```python
from build123d import *

# Parameters (mm, degrees)
ESQUISSE1_W                                        = 100
ESQUISSE1_H                                        = 150
BOSS_EXTRU_1_DEPTH                                 = 15
ESQUISSE2_W                                        = 25
ESQUISSE2_H                                        = 70
BOSS_EXTRU_2_DEPTH                                 = 60
ENL_V_MAT_EXTRU_1_DEPTH                            = 4.15
CHAMBRAGE_POUR_VIS_T_TE_RONDE_BOMB_E_M_D           = 3.4
CHAMBRAGE_POUR_VIS_T_TE_RONDE_BOMB_E_M_CBORE_D     = 7
CHAMBRAGE_POUR_VIS_T_TE_RONDE_BOMB_E_M_CBORE_DEPTH = 2.4
BOSS_EXTRU_3_DEPTH                                 = 10
CONG_1_R                                           = 7
CONG_2_R                                           = 2


with BuildPart() as part:
    # Esquisse1 → Boss.-Extru.1 (new body)
    with BuildSketch(Plane.XY):
        with Locations((50, 0)):
            Rectangle(ESQUISSE1_W, ESQUISSE1_H)
    extrude(amount=BOSS_EXTRU_1_DEPTH)

    # Esquisse2 → Boss.-Extru.2 (add)
    with BuildSketch(Plane.XY.offset(15)):
        with Locations((-12.5, 0)):
            Rectangle(ESQUISSE2_W, ESQUISSE2_H)
    extrude(amount=-BOSS_EXTRU_2_DEPTH)

    # Esquisse4 → Enlèv. mat.-Extru.1 (cut)
    with BuildSketch(Plane.ZY.offset(25)):
        with BuildLine():
            Line((-2.2, 0), (-2.2, 6.5))
            ThreePointArc((-2.2, 6.5), (-2.492893219, 7.207106781), (-3.2, 7.5))
            Line((-3.2, 7.5), (-9.7, 7.5))
            ThreePointArc((-9.7, 7.5), (-12.00671757, 7.13645949), (-14.089812398, 6.081081081))
            ThreePointArc((-14.089812398, 6.081081081), (-16.998209557, 4.607571798), (-20.218826659, 4.1))
            Line((-20.218826659, 4.1), (-33.7, 4.1))
            ThreePointArc((-33.7, 4.1), (-36.599137803, 2.899137803), (-37.8, 0))
            ThreePointArc((-37.8, 0), (-36.599137803, -2.899137803), (-33.7, -4.1))
            Line((-33.7, -4.1), (-20.218826659, -4.1))
            ThreePointArc((-20.218826659, -4.1), (-18.58641381, -4.22802272), (-16.993916418, -4.60896049))
            Line((-16.993916418, -4.60896049), (-16.993916418, -6.5))
            ThreePointArc((-16.993916418, -6.5), (-16.701023199, -7.207106781), (-15.993916418, -7.5))
            Line((-15.993916418, -7.5), (-9.7, -7.5))
            ThreePointArc((-9.7, -7.5), (-4.396699141, -5.303300859), (-2.2, 0))
        make_face()
    extrude(amount=-ENL_V_MAT_EXTRU_1_DEPTH, mode=Mode.SUBTRACT)

    # Chambrage pour vis à tête ronde bombée M32 (through all)
    with Locations(Plane(origin=(0, 0, -33.7), x_dir=(0, 0, 1), z_dir=(1, 0, 0))):
        with Locations((0, 0), (24, 0)):
            CounterBoreHole(CHAMBRAGE_POUR_VIS_T_TE_RONDE_BOMB_E_M_D / 2, CHAMBRAGE_POUR_VIS_T_TE_RONDE_BOMB_E_M_CBORE_D / 2, CHAMBRAGE_POUR_VIS_T_TE_RONDE_BOMB_E_M_CBORE_DEPTH)

    # Esquisse10 → Boss.-Extru.3 (add)
    with BuildSketch(Plane.XZ.offset(35)):
        Polygon((0, -45), (25, 0), (0, 0), align=None)
    boss_extru_3 = extrude(amount=-BOSS_EXTRU_3_DEPTH)

    # Symétrie1: Boss.-Extru.3 across plane
    add(boss_extru_3.mirror(Plane.ZX))

    # Congé1
    cong_1_edges = [part.edges().sort_by_distance(p)[0] for p in [
        (0, 35, 7.5),
        (0, -35, 7.5),
    ]]
    fillet(cong_1_edges, radius=CONG_1_R)

    # Congé2
    cong_2_edges = [part.edges().sort_by_distance(p)[0] for p in [
        (0, 0, 0),
        (100, -75, 7.5),
        (100, 75, 7.5),
        (0, -75, 7.5),
        (0, 75, 7.5),
    ]]
    fillet(cong_2_edges, radius=CONG_2_R)


solid = part.part
```
Geometry: final body of the model. Coordinates: model frame, mm. A direction names the side the tool comes from. Coordinates: 2 decimals unless noted, no trailing zeros. Loops run counter-clockwise (first coordinate to the right, second up) from the corner with the lowest first, then second, coordinate; pieces in that order, holes last. Notation, with made-up numbers: (76.25, -10) -> (130.25, -10) arc R25 cw to (130.25, 17) -> close; hole circle Ø9 at (64.5, 73.25). An arc over 180 degrees is marked (long way). Use a Markdown table: item, result. Add a question column.
(1) Section query A-A, the plane z = 11. Return loops of the section in (x, y), plus the area to 3 significant figures.
(2) Section query B-B, the plane y = 10. Return loops of the section in (x, z).
(3) Mould query, pull axis Z, two halves, no side actions, for faces 5 (the flat face through (100, -1, 7)), 6 (the flat face through (-13, 0, -45)), 7 (the cylindrical face through (-1.2, 2.1, -36.5)). Classes: pulls with the +Z half, pulls with the -Z half, needs draft (parallel to the pull), parting line crosses it, or undercut.
(4) Line query: line 1 along Y through (x, z) = (-0.9, -9.7); line 2 along Y through (x, z) = (-12.5, -9.7); line 3 along X through (y, z) = (-50.5, 0.5). Output: solid intervals per line, ascending.
(5) Pin query (flat end, axial travel): pin 1 Ø3.5 at (x, z) = (-22.5, -12.5) entering from +Y; pin 2 Ø4.5 at (y, z) = (64.5, 9) entering from -X; pin 3 Ø4 at (y, z) = (0, -33.7) entering from +X. Return the tip coordinate at first contact, or that it passes through.
(6) Section query D-D, the plane z = -22.5. Return loops of the section in (x, y), plus the area to 3 significant figures.
(7) Section query C-C, the plane x = 91. Return loops of the section in (y, z), plus the area to 3 significant figures.
(8) Access query for faces 1 (the flat face through (10, -25, -17)), 2 (the cylindrical face through (-22.954, -5.361, -4.455)), 3 (the flat face through (0, -58, 7)), 4 (the flat face through (-2.4, 2, -35)). Directions: +Z, -Z, +X, -X, +Y, -Y. A direction counts if a zero-diameter tool reaches every point of the face in a straight line with its end or side. Return the directions, or none.
Answer:
| question | item | result |
|---|---|---|
| 1 | outline | (-25, -35) -> (-7, -35) arc R7 cw to (0, -42) -> (0, -73) arc R2 ccw to (2, -75) -> (98, -75) arc R2 ccw to (100, -73) -> (100, 73) arc R2 ccw to (98, 75) -> (2, 75) arc R2 ccw to (0, 73) -> (0, 42) arc R7 cw to (-7, 35) -> (-25, 35) -> close |
| 1 | area | 16,800 mm^2 |
| 2 | outline | (-25, -45) -> (0, -45) -> (0, -2) arc R2 cw to (2, 0) -> (100, 0) -> (100, 15) -> (-25, 15) -> close |
| 3 | face 5 | needs draft |
| 3 | face 6 | pulls with the -Z half |
| 3 | face 7 | undercut |
| 4 | line 1 | y = -35 to -3.5, 3.5 to 35 |
| 4 | line 2 | y = -35 to -1.7, 1.7 to 35 |
| 4 | line 3 | x = 0 to 100 |
| 5 | pin 1 | stops at y = 35 |
| 5 | pin 2 | stops at x = 0 |
| 5 | pin 3 | stops at x = -2.4 |
| 6 | outline | (-25, -35) -> (12.5, -35) -> (12.5, -25) -> (0, -25) -> (0, 25) -> (12.5, 25) -> (12.5, 35) -> (-25, 35) -> (-25, 4.1) -> (-20.85, 4.1) -> (-20.85, -4.1) -> (-25, -4.1) -> close |
| 6 | area | 1,970 mm^2 |
| 7 | outline | (-75, 0) -> (75, 0) -> (75, 15) -> (-75, 15) -> close |
| 7 | area | 2,250 mm^2 |
| 8 | face 1 | -Z, +X |
| 8 | face 2 | -X |
| 8 | face 3 | +Z, -Z, -X, -Y |
| 8 | face 4 | +X |
